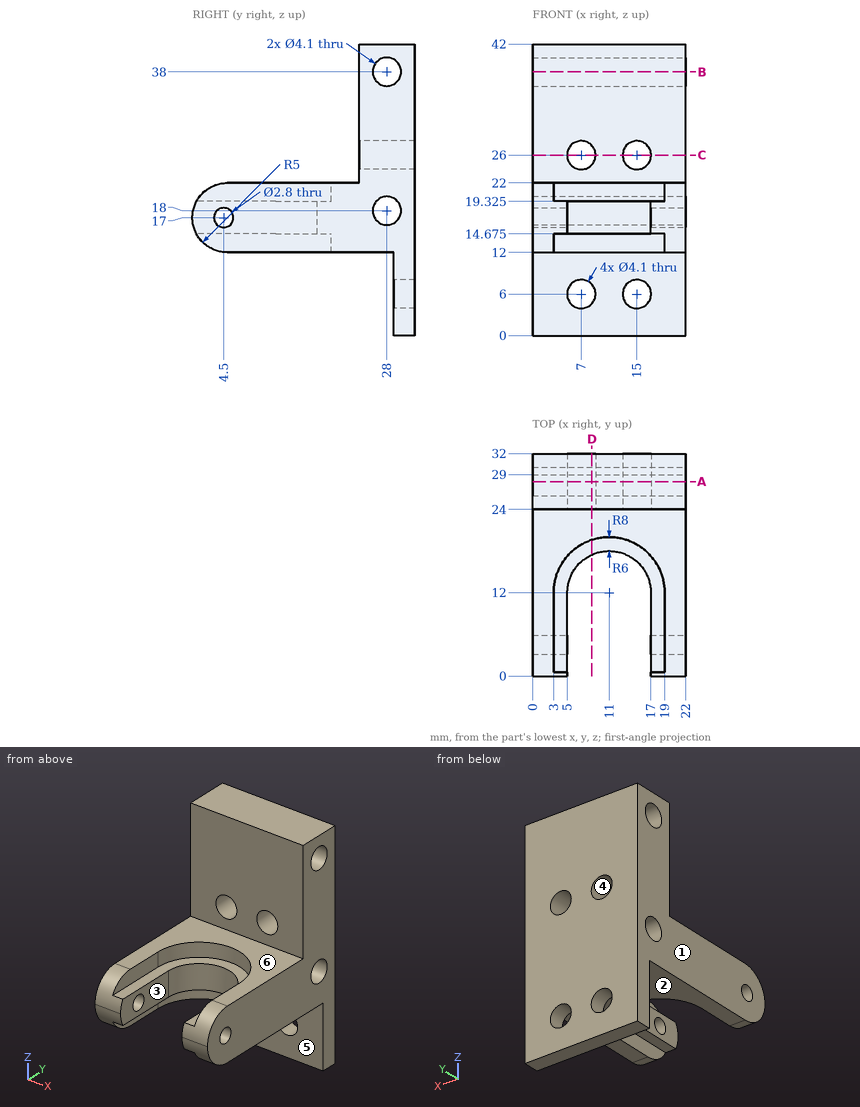
For this review, use the dimensioned drawing (mm, ordinates from the lowest corner) and the shaded views. A direction names the side the tool comes from. Give positions to 0.01 mm unless a question says otherwise; leave off trailing zeros. Write each loop counter-clockwise with the first axis right and the second up, starting at its lowest first coordinate (ties: lowest second). Pieces come first, ordered by that corner, then holes.
(1) For P1, Ø1.5, axis at x = 6.5, y = 20.5, coming from the +Z side; P2, Ø6, axis at x = 9, z = 7.5, coming from the -Y side; P3, Ø4.5, axis at x = 15, z = 26, coming from the -Y side, all flat-tipped, find the tip position at first contact; note any pin that passes through.
(2) Consider section B-B, the plane z = 38. Give the boundary of the cut face in (x, y).
(3) The part is to be moulded in two halves that separate along X. For the marked faces 1, 2 and 3, say which applies: released by +X, released by -X, zero draft, split by the parting line, or undercut.
(4) Tool access review of the marked faces 4, 5 and 6: name each direction out of +Z, -Z, +X, -X, +Y, -Y from which nothing blocks a thin tool from reaching the whole face with its end or side.
(5) Consider section D-D, the plane x = 8.5. Give the boundary of the cut face in (y, z) (3 decimals).
(6) Consider section C-C, the plane z = 26. Give the boundary of the cut face in (x, y).
(7) To check wall thickness, follow L1, parallel to X at y = 28, z = 26; L2, parallel to Z at x = 7, y = 30.9; L3, parallel to Z at x = 4.05, y = 4.5 (3 decimals). State the ranges of each line that lie inside material, in increasing order.
(8) Consider section A-A, the plane y = 28. Give the boundary of the cut face in (x, z).
Returned:
1. P1: stops at z = 22
1. P2: stops at y = 29
1. P3: stops at y = 24
2. outline: (0, 24) - (22, 24) - (22, 25.95) - (0, 25.95) - close; (0, 30.05) - (22, 30.05) - (22, 32) - (0, 32) - close
3. face 1: released by -X
3. face 2: zero draft
3. face 3: undercut
4. face 4: +Y, -Y
4. face 5: -Z, +X, -X, -Y
4. face 6: +Z, +X, -X, -Y
5. outline: (17.454, 14.675) - (19.599, 14.675) - (19.599, 12) - (29, 12) - (29, 7.397) - (32, 7.397) - (32, 24.603) - (24, 24.603) - (24, 22) - (19.599, 22) - (19.599, 19.325) - (17.454, 19.325) - close; (24, 27.397) - (32, 27.397) - (32, 42) - (24, 42) - close; (29, 0) - (32, 0) - (32, 4.603) - (29, 4.603) - close; hole circle Ø4.1 at (28, 18); hole circle Ø4.1 at (28, 38)
6. outline: (0, 24) - (4.95, 24) - (4.95, 32) - (0, 32) - close; (9.05, 24) - (12.95, 24) - (12.95, 32) - (9.05, 32) - close; (17.05, 24) - (22, 24) - (22, 32) - (17.05, 32) - close
7. L1: x = 0 to 4.95, 9.05 to 12.95, 17.05 to 22
7. L2: z = 0 to 3.95, 8.05 to 23.95, 28.05 to 42
7. L3: z = 14.675 to 15.6, 18.4 to 19.325
8. outline: (0, 12) - (22, 12) - (22, 15.95) - (0, 15.95) - close; (0, 20.05) - (22, 20.05) - (22, 35.95) - (0, 35.95) - close; (0, 40.05) - (22, 40.05) - (22, 42) - (0, 42) - close; hole circle Ø4.1 at (7, 26); hole circle Ø4.1 at (15, 26)
